from build123d import *

# Parameters (mm, degrees)
ENL_V_MAT_EXTRU_3_DEPTH      = 115.682169495
R_P_TITION_CIRCULAIRE1_COUNT = 17
ENL_V_MAT_EXTRU_4_DEPTH      = 115.682169495


with BuildPart() as part:
    # Esquisse1 → Révolution1 (revolve)
    with BuildSketch(Plane.XY, mode=Mode.PRIVATE) as r_volution1_sk:
        Polygon((-76, 40), (-76, 0), (-50, 0), (0, 0), (0, 40), (-50, 40), align=None)
    revolve(r_volution1_sk.sketch.rotate(Axis((0, 40, 0), (0, -1, 0)), 270), axis=Axis((0, 40, 0), (0, -1, 0)))

    # Esquisse5 → Enlèv. mat.-Extru.3 (cut, through all)
    with BuildSketch(Plane(origin=(0, 40, 0), x_dir=(1, 0, 0), z_dir=(0, 1, 0))):
        with BuildLine():
            ThreePointArc((-7.01239532, 75.675797398), (-17.400241796, 73.981292131), (-27.45436663, 70.867889435))
            Line((-27.45436663, 70.867889435), (-15.872453425, 55.785887304))
            Line((-15.872453425, 55.785887304), (-10.657472034, 57.012439782))
            Line((-10.657472034, 57.012439782), (-7.01239532, 75.675797398))
        make_face()
    enl_v_mat_extru_3 = extrude(amount=-ENL_V_MAT_EXTRU_3_DEPTH, mode=Mode.SUBTRACT)

    # Répétition circulaire1: Enlèv. mat.-Extru.3 ×17 about axis
    r_p_tition_circulaire1_axis = Axis((0, 0, 0), (0, 1, 0))
    for i in range(1, R_P_TITION_CIRCULAIRE1_COUNT):
        add(enl_v_mat_extru_3.rotate(r_p_tition_circulaire1_axis, i * 360 / R_P_TITION_CIRCULAIRE1_COUNT), mode=Mode.SUBTRACT)

    # Esquisse6 → Enlèv. mat.-Extru.4 (cut, through all)
    with BuildSketch(Plane(origin=(0, 40, 0), x_dir=(1, 0, 0), z_dir=(0, 1, 0))):
        with BuildLine():
            Line((-12.296722124, 3.175), (-15.496722124, 3.175))
            Line((-15.496722124, 3.175), (-15.496722124, -3.175))
            Line((-15.496722124, -3.175), (-12.296722124, -3.175))
            ThreePointArc((-12.296722124, -3.175), (12.7, 0), (-12.296722124, 3.175))
        make_face()
    extrude(amount=-ENL_V_MAT_EXTRU_4_DEPTH, mode=Mode.SUBTRACT)


solid = part.part
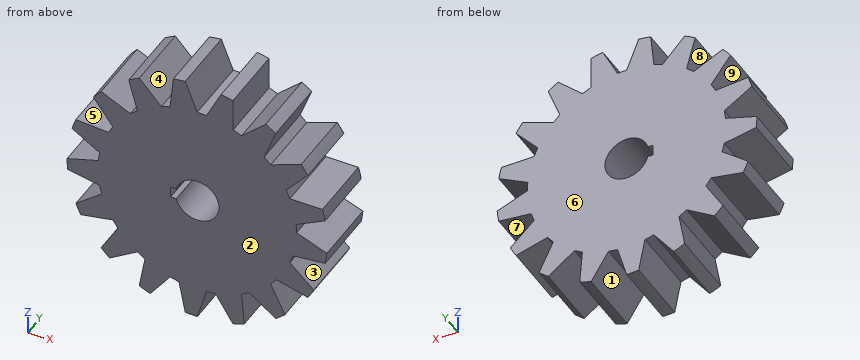
Work out the finished part from the listing and answer in its coordinate system (mm). Face numbers are marked on the shaded views. A direction names the side the tool comes from. Coordinates: 2 decimals unless noted, no trailing zeros. Loops run counter-clockwise (first coordinate to the right, second up) from the corner with the lowest first, then second, coordinate; pieces in that order, holes last. Notation, with made-up numbers: (36, 81.5) -> (72, 81.5) arc R20 ccw to (72, 114.5) -> close; hole circle Ø4 at (48.25, 12). An arc over 180 degrees is marked (long way). Answer as CSV lines item,"result".
1) Flat-ended cylindrical pins translate along their axes: pin 1 (5 mm diameter, centred on x = 59, z = -42, fed in from -Y); pin 2 (2.5 mm diameter, centred on x = -13, y = 25, fed in from +Z); pin 3 (12 mm diameter, centred on x = -58.5, y = 23.5, fed in from -Z); pin 4 (12 mm diameter, centred on y = 16.5, z = 40, fed in from +X). Find the tip coordinate at first contact, or state that the pin passes through.
A:
pin 1,"passes through"
pin 2,"stops at z = 75.09"
pin 3,"stops at z = -54.95"
pin 4,"stops at x = 64.62"
2) The part is cut by section B-B (z = 48.5). Give the vertices of the cut face in (x, y).
A:
outline,"(-58.51, 0) -> (-50.63, 0) -> (-50.63, 40) -> (-58.51, 40) -> close; (-35.56, 0) -> (41.21, 0) -> (41.21, 40) -> (-35.56, 40) -> close"
3) The part is cut by section A-A (z = -54). Give the vertices of the cut face in (x, y), and give its area (3 significant figures).
A:
outline,"(-53.48, 0) -> (-47.64, 0) -> (-47.64, 40) -> (-53.48, 40) -> close; (-31.37, 0) -> (26.03, 0) -> (26.03, 40) -> (-31.37, 40) -> close; (36.85, 0) -> (50.14, 0) -> (50.14, 40) -> (36.85, 40) -> close"
area,"3,060 mm²"
4) For a pull along X with two mould halves and no side action, classify the marked faces 6, 7, 8 and 9 as released by +X, released by -X, zero draft, split by the parting line, or undercut.
A:
face 6,"zero draft"
face 7,"released by +X"
face 8,"undercut"
face 9,"released by -X"
5) Straight lines are drawn through the part: probe 1 along X at (y, z) = (8, 67.5); probe 2 along Z at (x, y) = (62.5, 35.5); probe 3 along X at (y, z) = (35, 56). For each, find the intervals that lie inside material, in ascending order.
A:
probe 1,"x = -34.92 to -33.38, -14.69 to -3.77, 10.3 to 20.84"
probe 2,"z = -39.43 to -28.75, -15.2 to -1.79, 7.76 to 20.88, 37.65 to 43.24"
probe 3,"x = -37.63 to -22.73, -15.85 to 20.94, 30.4 to 44.04"
6) For the marked faces 1, 2, 3, 4 and 5, determine the directions among +Z, -Z, +X, -X, +Y, -Y from which every point of the face is accessible in a straight line to the end or side of a thin tool.
A:
face 1,"-Z, +Y, -Y"
face 2,"+Z, -Z, +X, -X, -Y"
face 3,"+X, +Y, -Y"
face 4,"+Z, +Y, -Y"
face 5,"+Y, -Y"
